The model under review builds one solid part; all positions refer to its coordinate system, in mm. A direction names the side the tool comes from. Round coordinates to 2 decimals unless told otherwise and drop trailing zeros. Order: outer loops, then holes, each group sorted by start corner. A loop starts at its lowest first (then second) coordinate and runs counter-clockwise, first axis right, second up. Notation, with made-up numbers: M 33.5,83 L 77.5,83 A13 ccw 77.5,104 Z; hole C 41.5,12 d4. An arc over 180 degrees is marked long. Answer as CSV lines item,"result". Start each with the question number.
from build123d import *

# Parameters (mm, degrees)
ESQUISSE1_R             = 5.5
BASE_EXTRUSION_DEPTH    = 16
ESQUISSE2_R             = 3
BOSS_EXTRU_1_DEPTH      = 2
ESQUISSE3_R             = 8
BOSS_EXTRU_2_DEPTH      = 1.5
ESQUISSE4_R             = 6.5
BOSS_EXTRU_3_DEPTH      = 7
ESQUISSE5_R             = 4.5
ENL_V_MAT_EXTRU_1_DEPTH = 19
ESQUISSE6_W             = 3
ESQUISSE6_H             = 4
ENL_V_MAT_EXTRU_2_DEPTH = 1.5
ENL_V_MAT_EXTRU_2_TAPER = 5
BOSS_EXTRU_4_DEPTH      = 2
ENL_V_MAT_EXTRU_3_REACH = 17
ESQUISSE8_R             = 1.5
ESQUISSE9_R             = 1.5
ENL_V_MAT_EXTRU_4_DEPTH = 27.5000001
CONG_2_R                = 0.25


with BuildPart() as part:
    # Esquisse1 → Base-Extrusion (new body)
    with BuildSketch(Plane.XY):
        Circle(ESQUISSE1_R)
    extrude(amount=BASE_EXTRUSION_DEPTH)

    # Esquisse2 → Boss.-Extru.1 (add)
    with BuildSketch(Plane.XY.offset(16)):
        Circle(ESQUISSE2_R)
    extrude(amount=BOSS_EXTRU_1_DEPTH)

    # Esquisse3 → Boss.-Extru.2 (add)
    with BuildSketch(Plane(origin=(0, 0, 0), x_dir=(-1, 0, 0), z_dir=(0, 0, -1))):
        Circle(ESQUISSE3_R)
    extrude(amount=BOSS_EXTRU_2_DEPTH)

    # Esquisse4 → Boss.-Extru.3 (add)
    with BuildSketch(Plane(origin=(0, 0, -1.5), x_dir=(-1, 0, 0), z_dir=(0, 0, -1))):
        Circle(ESQUISSE4_R)
    extrude(amount=BOSS_EXTRU_3_DEPTH)

    # Esquisse5 → Enlèv. mat.-Extru.1 (cut)
    with BuildSketch(Plane(origin=(0, 0, -8.5), x_dir=(-1, 0, 0), z_dir=(0, 0, -1))):
        Circle(ESQUISSE5_R)
    extrude(amount=-ENL_V_MAT_EXTRU_1_DEPTH, mode=Mode.SUBTRACT)

    # Esquisse6 → Enlèv. mat.-Extru.2 (cut)
    with BuildSketch(Plane(origin=(0, 0, -8.5), x_dir=(-1, 0, 0), z_dir=(0, 0, -1))):
        with Locations((0, 5)):
            Rectangle(ESQUISSE6_W, ESQUISSE6_H)
    extrude(amount=-ENL_V_MAT_EXTRU_2_DEPTH, taper=ENL_V_MAT_EXTRU_2_TAPER, mode=Mode.SUBTRACT)

    # Esquisse7 → Boss.-Extru.4 (add)
    with BuildSketch(Plane(origin=(0, -5, 0), x_dir=(-1, 0, 0), z_dir=(0, 1, 0))):
        with BuildLine():
            Line((3, -5), (3, -1.5))
            Line((3, -1.5), (-3, -1.5))
            Line((-3, -1.5), (-3, -5))
            ThreePointArc((-3, -5), (0, -8), (3, -5))
        make_face()
    extrude(amount=-BOSS_EXTRU_4_DEPTH)

    # Esquisse8 → Enlèv. mat.-Extru.3 (cut, up to next)
    with BuildSketch(Plane.XZ.offset(7), mode=Mode.PRIVATE) as enl_v_mat_extru_3_sk1:
        with Locations((0, -5)):
            Circle(ESQUISSE8_R)
    enl_v_mat_extru_3_tool1 = extrude(enl_v_mat_extru_3_sk1.sketch, amount=-ENL_V_MAT_EXTRU_3_REACH, mode=Mode.PRIVATE) & part.part
    add(enl_v_mat_extru_3_tool1.solids().sort_by_distance((0, -7, -5))[0], mode=Mode.SUBTRACT)

    # Esquisse9 → Enlèv. mat.-Extru.4 (cut, through all)
    with BuildSketch(Plane.XY.offset(18)):
        Circle(ESQUISSE9_R)
    extrude(amount=-ENL_V_MAT_EXTRU_4_DEPTH, mode=Mode.SUBTRACT)

    # Congé2
    cong_2_edges = [part.edges().sort_by_distance(p)[0] for p in [
        (8, 0, 0),
        (8, 0, -1.5),
    ]]
    fillet(cong_2_edges, radius=CONG_2_R)


solid = part.part
Item 1: The part is to be moulded in two halves that separate along Y. For faces 1 (the cylindrical face through (-1.5, -5.64, -4.93)), 2 (the cylindrical face through (-3, 0, 17)), 3 (the flat face through (0, -2, 10.5)), say which applies: +Y half, -Y half, draft (parallel to the pull), parting line (faces both ways), or undercut.
Item 2: Consider section B-B (x = 0). State how many separate pieces and enclosed holes the cut face has, and give its area (3 significant figures).
Item 3: Tool access review of faces 4 (the cylindrical face through (0.07, -6.65, -8)), 5 (the flat face through (-3, -6, -3)), 6 (the flat face through (3, -6, -3)), 7 (the flat face through (0, 5, -7)): name each direction out of +Z, -Z, +X, -X, +Y, -Y from which nothing blocks a thin tool from reaching the whole face with its end or side.
Item 4: Consider section D-D (z = 14.75). State the section outline as (x, y) points, and give its area (3 significant figures).
Item 5: Consider section C-C (z = 5.5). State the section outline as (x, y) points.
Item 6: Wall thickness on probe 1 along Y at (x, z) = (0, 15.25); probe 2 along Y at (x, z) = (0, -0.5); probe 3 along Z at (x, y) = (-5.5, -5.5): over which ranges is each line inside the solid? List them lowest first. Write a range as [from, to].
Item 7: For pin 1 (1.8 mm diameter, centred on x = 0, y = 5.5, fed in from -Z); pin 2 (2.5 mm diameter, centred on x = 0, y = 0, fed in from -Z); pin 3 (5 mm diameter, centred on x = 0, z = -5, fed in from -Y); pin 4 (4 mm diameter, centred on y = -1, z = 8.5, fed in from -X), all flat-tipped, find the tip position at first contact; note any pin that passes through.
Item 8: Consider section A-A (y = 0). State the section outline as (x, z) points, and give its area (3 significant figures).
Reported:
1,face 1,"draft"
1,face 2,"parting line"
1,face 3,"undercut"
2,separate pieces,"3"
2,enclosed holes,"0"
2,area,"102 mm²"
3,face 4,"-Z, -Y"
3,face 5,"-Z, -X, -Y"
3,face 6,"-Z, +X, -Y"
3,face 7,"-Z, +Y"
4,outline,"C 0,0 d11; hole C 0,0 d3"
4,area,"88.0 mm²"
5,outline,"C 0,0 d11; hole C 0,0 d9"
6,probe 1,"y = [-5.5, -1.5], [1.5, 5.5]"
6,probe 2,"y = [-8, -4.5], [4.5, 8]"
6,probe 3,"z = [-1.5, 0]"
7,pin 1,"stops at z = -7"
7,pin 2,"passes through"
7,pin 3,"stops at y = -7"
7,pin 4,"stops at x = -5.5"
8,outline,"M -8,-1.25 A0.25 ccw -7.75,-1.5 L -6.5,-1.5 L -6.5,-8.5 L -4.5,-8.5 L -4.5,10.5 L -1.5,10.5 L -1.5,18 L -3,18 L -3,16 L -5.5,16 L -5.5,0 L -7.75,0 A0.25 ccw -8,-0.25 Z; M 1.5,10.5 L 4.5,10.5 L 4.5,-8.5 L 6.5,-8.5 L 6.5,-1.5 L 7.75,-1.5 A0.25 ccw 8,-1.25 L 8,-0.25 A0.25 ccw 7.75,0 L 5.5,0 L 5.5,16 L 3,16 L 3,18 L 1.5,18 Z"
8,area,"109 mm²"
